Part model, mm, in its own coordinate system. A direction names the side the tool comes from. Coordinates: 2 decimals unless noted, no trailing zeros. Write each loop counter-clockwise with the first axis right and the second up, starting at its lowest first coordinate (ties: lowest second). Pieces come first, ordered by that corner, then holes. Notation, with made-up numbers: (-2, -16.5) -> (38, -16.5) arc R28 ccw to (38, 4.5) -> close; hole circle Ø6 at (66, -19.75). An arc over 180 degrees is marked (long way). Write item = value, one per line. Start each with the question number.
Q1. Band-saw the part on A-A, the plane z = 0. List the corners of the cut face in (x, y) (3 decimals).
Q2. Probe line 1 (Y direction, x = 1.45, z = -12.5); line 2 (Y direction, x = 1.7, z = -14.5); line 3 (Y direction, x = 0.3, z = 33). List the from-to ranges inside material, lowest first.
Q3. Band-saw the part on B-B, the plane y = 9. List the corners of the cut face in (x, z) (3 decimals).
Q4. Pin check, flat tips, straight feed: P1, Ø1, axis at x = 1.5, y = -54, coming from the +Z side (3 decimals); P2, Ø3, axis at y = -8.73, z = -13.49, coming from the -X side; P3, Ø1.6, axis at x = 1.5, y = -55.5, coming from the -Z side (3 decimals). Stop position of each tip, or through.
Q5. Tool access for faces 5 (the cylindrical face through (0.87, 28.266, 24.222)), 6 (the flat face through (2, 13, -28.575)): list every direction of +Z, -Z, +X, -X, +Y, -Y with a clear straight run to the whole face (end or side of a thin tool).
Q6. Pull direction Z, two halves, no side cores. Call faces 1 (the conical face through (1.4, 59.93, 43.12)), 2 (the flat face through (2, 35.719, 38)), 3 (the conical face through (1.244, -24.621, -1.002)), 4 (the cylindrical face through (1.61, -37.617, 44.909)): released by +Z, released by -Z, zero draft, split by the parting line, or undercut.
Autodesk Inventor part; units mm, degrees
ref_plane "YZ Plane" through (0, 0, 0) normal (1, 0, 0) x (0, 1, 0)
ref_plane "XZ Plane" through (0, 0, 0) normal (0, 1, 0) x (-1, 0, 0)
ref_plane "XY Plane" through (0, 0, 0) normal (0, 0, 1) x (1, 0, 0)
sketch "Sketch1" plane through (0, 0, 0) normal (1, 0, 0) x (0, 1, 0)
  line L0 (-73.8187, -28.575) -> (73.8188, -28.575)
  line L1 (73.8188, -28.575) -> (73.8187, 28.575)
  line L2 (73.8187, 28.575) -> (-73.8188, 28.575)
  line L3 (-73.8188, 28.575) -> (-73.8187, -28.575)
  line L4 (-73.8187, -28.575) -> (73.8187, 28.575) construction
  line L5 (73.8188, -28.575) -> (-73.8188, 28.575) construction
  line L6 (-73.8187, 0) -> (73.8188, 0) construction
  line L7 (-8.7312, -47.625) -> (-40.4812, -47.625)
  line L8 (-40.4812, -47.625) -> (-40.4812, 47.625)
  line L9 (-40.4812, 47.625) -> (-8.7312, 47.625)
  line L10 (-8.7312, 47.625) -> (-8.7312, -47.625)
  line L11 (-8.7312, -47.625) -> (-40.4812, 47.625) construction
  line L12 (-40.4812, -47.625) -> (-8.7312, 47.625) construction
  circle A0 centre (-30.9563, 38.1) radius 9.525 construction
  circle A1 centre (-30.9563, 38.1) radius 1.7526
  circle A2 centre (-30.9563, -38.1) radius 1.7526
  line L13 (35.7188, 47.625) -> (73.8188, 47.625)
  line L14 (73.8188, 47.625) -> (73.8188, -47.625)
  line L15 (73.8188, -47.625) -> (35.7188, -47.625)
  line L16 (35.7188, -47.625) -> (35.7188, 47.625)
  line L17 (35.7188, 47.625) -> (73.8188, -47.625) construction
  line L18 (73.8188, 47.625) -> (35.7188, -47.625) construction
  line L19 (86.5188, -9.525) -> (61.1188, -9.525)
  line L20 (61.1188, -9.525) -> (61.1188, 9.525)
  line L21 (61.1188, 9.525) -> (86.5188, 9.525)
  line L22 (86.5188, 9.525) -> (86.5188, -9.525)
  line L23 (86.5188, -9.525) -> (61.1188, 9.525) construction
  line L24 (61.1188, -9.525) -> (86.5188, 9.525) construction
  point P0 (0, 0)
  point P1 (-24.6062, 0)
  point P2 (-8.7312, -28.575)
  point P3 (-40.4812, -28.575)
  point P4 (-40.4812, 28.575)
  point P5 (-8.7312, 28.575)
  point P6 (54.7687, 0)
  point P7 (35.7188, -28.575)
  point P8 (35.7187, 28.575)
  point P9 (73.8187, -9.525)
  point P10 (73.8187, 9.525)
  dimension "d0" = 147.6375
  dimension "d1" = 57.15
  dimension "d4" = 33.3375
  dimension "d5" = 31.75
  dimension "d6" = 19.05
  dimension "d7" = 3.5052
  dimension "d34" = 38.1
  dimension "d35" = 95.25
  dimension "d36" = 25.4
  dimension "d37" = 19.05
extrude "Extrusion1" add sketch "Sketch1" along normal blind 3.175 contours L3 L2 L8 L0 | L8 L2 L10 L0 | L0 L10 L7 L8 | L10 L2 L16 L0 | L8 L9 L10 L2 | L16 L2 L1 L21 L20 L19 L0 | L0 L14 L15 L16 | L16 L13 L14 L2
fillet "Fillet1" radius 9.525 2 edges at (1.5875, -40.4812, 47.625) (1.5875, -40.4812, -47.625)
fillet "Fillet2" radius 6.35 12 edges at (1.5875, -40.4812, 28.575) (1.5875, -40.4812, -28.575) (1.5875, -8.7312, -28.575) (1.5875, -8.7312, 28.575) (1.5875, 35.7188, -28.575) (1.5875, 35.7188, -47.625) (1.5875, 35.7188, 47.625) (1.5875, 35.7187, 28.575) (1.5875, 61.1188, 9.525) (1.5875, 73.8187, 9.525) (1.5875, 61.1188, -9.525) (1.5875, 73.8187, -9.525)
fillet "Fillet3" radius 12.7 2 edges at (1.5875, -73.8187, -28.575) (1.5875, -73.8188, 28.575)
chamfer "Chamfer3" distance 12.7 angle 45 2 edges at (1.5875, -8.7312, -47.625) (1.5875, -8.7312, 47.625)
sketch "Sketch2" plane through (3.175, 0, 0) normal (1, 0, 0) x (0, 0, -1)
  point P0 (-23.0187, 48.4188)
  point P1 (-23.0187, 42.0688)
  point P2 (-23.0187, 35.7188)
  point P3 (-23.0187, 29.3688)
  point P4 (23.0188, 48.4188)
  point P5 (23.0188, 42.0688)
  point P6 (23.0188, 35.7188)
  point P7 (23.0188, 29.3688)
  point P8 (13.4938, -8.7312)
  point P9 (13.4938, -15.0812)
  point P10 (-13.4937, -8.7312)
  point P11 (-13.4937, -15.0812)
hole "Hole1" at (3.175, 48.4188, 23.0187) at (3.175, 42.0688, 23.0187) at (3.175, 35.7188, 23.0187) at (3.175, 29.3688, 23.0187) at (3.175, 48.4188, -23.0188) at (3.175, 42.0688, -23.0188) at (3.175, 35.7188, -23.0188) at (3.175, 29.3688, -23.0188) at (3.175, -8.7312, -13.4938) at (3.175, -15.0812, -13.4938) at (3.175, -8.7312, 13.4937) at (3.175, -15.0812, 13.4937) direction (-1, 0, 0) diameter 3.2639 end through all countersink diameter 5.715 countersink angle 82
sketch "Sketch3" plane through (3.175, 0, 0) normal (1, 0, 0) x (0, 0, -1)
  point P0 (0, -26.1937)
  point P1 (9.525, -26.1937)
  point P2 (9.525, -64.2937)
  point P3 (0, -64.2937)
hole "Hole2" at (3.175, -26.1937, 0) at (3.175, -26.1937, -9.525) at (3.175, -64.2937, -9.525) at (3.175, -64.2937, 0) direction (-1, 0, 0) diameter 3.5052 end through all countersink diameter 7.0866 countersink angle 82
fillet "Fillet4" radius 1.5875 2 edges at (1.5875, 73.8188, 47.625) (1.5875, 73.8188, -47.625)
sketch "Sketch4" plane through (3.175, 0, 0) normal (1, 0, 0) x (0, 0, -1)
  point P0 (33.3375, 57.9438)
  point P1 (42.8625, 57.9438)
  point P2 (42.8625, 45.2438)
  point P3 (33.3375, 45.2438)
  point P4 (-42.8625, 45.2438)
  point P5 (-33.3375, 45.2438)
  point P6 (-33.3375, 57.9438)
  point P7 (-42.8625, 57.9438)
hole "Hole3" at (3.175, 57.9438, -33.3375) at (3.175, 57.9438, -42.8625) at (3.175, 45.2438, -42.8625) at (3.175, 45.2438, -33.3375) at (3.175, 45.2438, 42.8625) at (3.175, 45.2438, 33.3375) at (3.175, 57.9438, 33.3375) at (3.175, 57.9438, 42.8625) direction (-1, 0, 0) diameter 3.7973 end through all countersink diameter 7.0866 countersink angle 82
properties part number "Bottom Plate" material "UHMW, White"
Ans:
q1.outline = (0, -73.819) -> (3.175, -73.819) -> (3.175, -67.837) -> (1.115, -66.046) -> (0, -66.046) -> close; (0, -62.541) -> (1.115, -62.541) -> (3.175, -60.75) -> (3.175, -29.737) -> (1.115, -27.946) -> (0, -27.946) -> close; (0, -24.441) -> (1.115, -24.441) -> (3.175, -22.65) -> (3.175, 61.119) -> (0, 61.119) -> close
q2.line_1 = -73.82 to -16.38, -13.79 to -10.03, -7.44 to 72.85
q2.line_2 = -73.82 to -16.37, -13.8 to -10.02, -7.45 to 73.67
q2.line_3 = -40.78 to -8.43, 35.42 to 43.38, 47.11 to 56.08, 59.81 to 73.82
q3.outline = (0, -28.575) -> (3.175, -28.575) -> (3.175, 28.575) -> (0, 28.575) -> close
q4.P1 = 28.575
q4.P2 = through
q4.P3 = -28.575
q5.face_5 = +X, -X
q5.face_6 = -Z, +X, -X
q6.face_1 = undercut
q6.face_2 = zero draft
q6.face_3 = undercut
q6.face_4 = released by +Z
